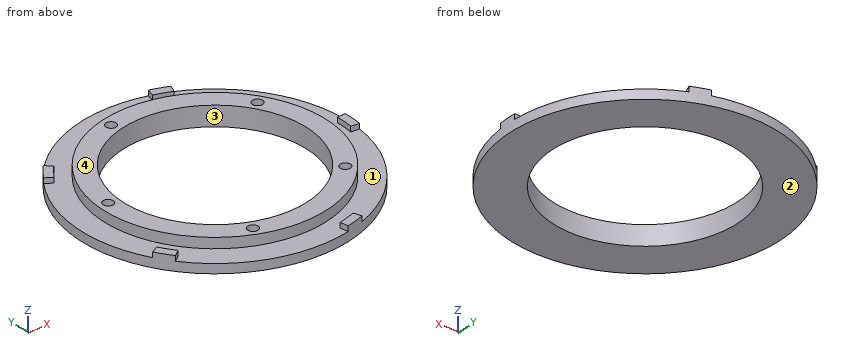
Autodesk Fusion 360 part; units mm, degrees
sketch "Sketch1" plane through (0, 0, 0) normal (0, 0, 1) x (1, 0, 0)
  circle A0 centre (0, 0) radius 65
  circle A1 centre (0, 0) radius 44.5
  circle A2 centre (0, 0) radius 54
  line L0 (44.5, 30.59) -> (44.5, 0) construction
  line L1 (-10.3681, 43.2753) -> (-10.3681, 52.9953) construction
  circle A3 centre (-10.3681, 48.1353) radius 2.5
  circle A4 centre (-48.9833, 5.014) radius 2.5
  circle A5 centre (-19.9052, -45.0365) radius 2.5
  circle A6 centre (36.6812, -32.8481) radius 2.5
  circle A7 centre (42.5755, 24.7353) radius 2.5
  line L2 (0, 0) -> (65, 0) construction
  line L3 (0, 0) -> (65, 0) construction
  line L4 (18.85, 58.0144) -> (20.0861, 61.8187)
  line L5 (26.7406, 54.8264) -> (28.4941, 58.4216)
  line L6 (-49.35, 35.8549) -> (-52.5861, 38.206)
  line L7 (-43.8797, 42.3742) -> (-46.7571, 45.1528)
  line L8 (-49.35, -35.8549) -> (-52.5861, -38.206)
  line L9 (-53.8598, -28.6378) -> (-57.3916, -30.5157)
  line L10 (18.85, -58.0144) -> (20.0861, -61.8187)
  line L11 (10.5925, -60.0733) -> (11.2871, -64.0125)
  line L12 (61, 0) -> (65, 0)
  line L13 (60.4064, -8.4896) -> (64.3674, -9.0463)
  arc A8 (26.7406, 54.8264) -> (18.85, 58.0144) centre (0, 0) ccw
  arc A9 (60.4064, -8.4896) -> (61, 0) centre (0, 0) ccw
  arc A10 (-43.8797, 42.3742) -> (-49.35, 35.8549) centre (0, 0) ccw
  arc A11 (-53.8598, -28.6378) -> (-49.35, -35.8549) centre (0, 0) ccw
  arc A12 (10.5925, -60.0733) -> (18.85, -58.0144) centre (0, 0) ccw
  line L14 (0, 0) -> (42.5755, 24.7353) construction
  line L15 (0, 0) -> (0, -65) construction
  dimension "d1" = 130
  dimension "d2" = 89
  dimension "d3" = 108
  dimension "d4" = 5
  dimension "d6" = 360
  dimension "d11" = 360
  dimension "d22" = 30.156
  dimension "d23" = 61
  dimension "d24" = 10
  dimension "d26" = 18
extrude "Extrude1" add sketch "Sketch1" along normal blind 7 contours A0 L12 L13 A9 | A0 L4 L5 A8 | A0 L10 L11 A12 | A0 L6 L7 A10 | A0 L8 L9 A11 makes body 1 at (64.8749, -4.0311, 4.6667) makes body 2 at (21.9942, 61.1658, 4.6667) makes body 3 at (16.2137, -62.9453, 4.6667) makes body 4 at (-51.9871, 39.0172, 4.6667) makes body 5 at (-53.1725, -37.3857, 4.6667)
extrude "Extrude2" add sketch "Sketch1" along normal blind 4.5 contours A0 L4 L5 L6 L7 L8 L9 L10 L11 L12 L13 A8 A9 A10 A11 A12 bodies 1 2 3 4 5
extrude "Extrude3" add sketch "Sketch1" along normal blind 9.5 contours A2 bodies 1
extrude "Extrude4" add sketch "Sketch1" along normal blind 1.5 contours A3 | A4 | A5 | A6 | A7 bodies 1
Read the model definition and answer for the solid it produces. Units are mm, in the model's axes. Face numbers are marked on the shaded views. A direction names the side the tool comes from. Round coordinates to 2 decimals unless told otherwise and drop trailing zeros. Write each loop counter-clockwise with the first axis right and the second up, starting at its lowest first coordinate (ties: lowest second). Pieces come first, ordered by that corner, then holes. Notation, with made-up numbers: (87.25, 17) -> (113.25, 17) arc R11 ccw to (113.25, 27) -> close; hole circle Ø4 at (73, 14). An arc over 180 degrees is marked (long way). Answer in a Markdown table with one row per item. Add a question column.
1) Find section B-B, the plane x = 36. Determine the outline of the cut face in (y, z).
2) Consider line 1 (Y direction, x = 0, z = 3.25); line 2 (Y direction, x = 41, z = 6.75); line 3 (Y direction, x = 35, z = 4). Determine where each line is inside the solid, lowest interval first.
3) Determine the mould class of the marked faces 3 and 4 for opening direction Y: pulls with the +Y half, pulls with the -Y half, needs draft (parallel to the pull), parting line crosses it, or undercut.
4) Which of the six approach directions +Z, -Z, +X, -X, +Y, -Y give full straight-line access (tool end or side, diameter ignored) to the marked faces 1 and 2?
5) Find section A-A, the plane x = 0. Determine the outline of the cut face in (y, z).
6) Given P1, Ø1.5, axis at y = -35, z = 7.5, coming from the -X side; P2, Ø3, axis at x = -40.5, z = 2.5, coming from the +Y side; P3, Ø5.5, axis at x = -10, y = 49, coming from the +Z side; P4, Ø7, axis at x = -48, y = 42.5, coming from the +Z side, each flat-ended and moving along its own axis, determine where each tip first touches the part or whether it passes through.
Findings below:
| question | item | result |
|---|---|---|
| 1 | outline | (-54.12, 0) -> (-26.16, 0) -> (-26.16, 9.5) -> (-30.44, 9.5) -> (-30.44, 1.5) -> (-35.25, 1.5) -> (-35.25, 9.5) -> (-40.25, 9.5) -> (-40.25, 4.5) -> (-54.12, 4.5) -> close; (26.16, 0) -> (54.12, 0) -> (54.12, 4.5) -> (40.25, 4.5) -> (40.25, 9.5) -> (26.16, 9.5) -> close |
| 2 | line 1 | -65 to -44.5, 44.5 to 65 |
| 2 | line 2 | -35.14 to -17.3, 17.3 to 22.79, 26.68 to 35.14 |
| 2 | line 3 | -54.77 to -34.7, -31 to -27.48, 27.48 to 54.77 |
| 3 | face 3 | undercut |
| 3 | face 4 | needs draft |
| 4 | face 1 | +Z |
| 4 | face 2 | -Z, +X, -X, +Y, -Y |
| 5 | outline | (-65, 0) -> (-44.5, 0) -> (-44.5, 9.5) -> (-54, 9.5) -> (-54, 4.5) -> (-65, 4.5) -> close; (44.5, 0) -> (65, 0) -> (65, 4.5) -> (54, 4.5) -> (54, 9.5) -> (44.5, 9.5) -> close |
| 6 | P1 | x = -55.13 |
| 6 | P2 | y = 52 |
| 6 | P3 | z = 9.5 |
| 6 | P4 | z = 7 |
